from build123d import *

# Parameters (mm, degrees)
SKETCH2_R           = 50
SKETCH2_R_2         = 30
BOSS_EXTRUDE1_DEPTH = 25
SKETCH3_W           = 66
SKETCH3_H           = 13
CUT_EXTRUDE1_DEPTH  = 25


with BuildPart() as part:
    # Sketch2 → Boss-Extrude1 (new body)
    with BuildSketch(Plane(origin=(0, 0, 0), x_dir=(1, 0, 0), z_dir=(0, 1, 0))):
        with Locations(Location((0, 0, 0), (0, 0, 270))):
            Circle(SKETCH2_R)
        with Locations(Location((0, 0, 0), (0, 0, 270))):
            Circle(SKETCH2_R_2, mode=Mode.SUBTRACT)
    extrude(amount=BOSS_EXTRUDE1_DEPTH)

    # Sketch3 → Cut-Extrude1 (cut)
    with BuildSketch(Plane(origin=(0, 25, 0), x_dir=(1, 0, 0), z_dir=(0, 1, 0))):
        with Locations((0, 1.5)):
            Rectangle(SKETCH3_W, SKETCH3_H)
    extrude(amount=-CUT_EXTRUDE1_DEPTH, mode=Mode.SUBTRACT)


solid = part.part
Could you check a few things on this model? Use its own coordinates, in mm. A direction names the side the tool comes from. Give positions to 0.01 mm unless a question says otherwise; leave off trailing zeros. Order: outer loops, then holes, each group sorted by start corner. A loop starts at its lowest first (then second) coordinate and runs counter-clockwise, first axis right, second up.
1. Suppose I cut it at D-D (x = 40). List the corners of the cut face in (y, z) for me, plus the area to 3 significant figures.
2. Suppose I cut it at B-B (z = 0). List the corners of the cut face in (x, y) for me, plus the area to 3 significant figures.
3. Will these pins go through, and if not, where does the flat tip stop? P1, Ø1.7, axis at x = -32, y = 15, coming from the -Z side; P2, Ø2, axis at x = 30, y = 15.5, coming from the +Z side; P3, Ø12, axis at x = -8, y = 15.5, coming from the +Z side; P4, Ø10, axis at x = 26.5, z = -7.5, coming from the +Y side.
4. Suppose I cut it at A-A (x = 0). List the corners of the cut face in (y, z) for me, plus the area to 3 significant figures.
5. For faces 1 (the flat face through (-22, 0, 22)), 2 (the flat face through (-33, 13, -1)), which set-ups out of +Z, -Z, +X, -X, +Y, -Y let a thin tool reach every point of the face, with its end or its side?
6. Suppose I cut it at C-C (y = 21). List the corners of the cut face in (x, z) for me.
7. I need wall thicknesses on L1, parallel to X at y = 18.75, z = 18; L2, parallel to X at y = 21, z = -25.5; L3, parallel to Z at x = 19, y = 19. Which ranges of each line are inside material? Lowest first, please.
8. We'd pull the mould along Z, two halves only. Please class faces 3 (the cylindrical face through (15.02, 12.32, 47.69)), 4 (the flat face through (31, 13, 5)), 5 (the flat face through (-22, 25, 22)): pulls with the +Z half, pulls with the -Z half, needs draft (parallel to the pull), parting line crosses it, or undercut.
Solved:
1. outline: (0, -30) - (25, -30) - (25, 30) - (0, 30) - close
1. area: 1,500 mm2
2. outline: (-50, 0) - (-33, 0) - (-33, 25) - (-50, 25) - close; (33, 0) - (50, 0) - (50, 25) - (33, 25) - close
2. area: 850 mm2
3. P1: stops at z = -39.11
3. P2: stops at z = 40.73
3. P3: stops at z = 49.96
3. P4: stops at y = 25
4. outline: (0, -50) - (25, -50) - (25, -30) - (0, -30) - close; (0, 30) - (25, 30) - (25, 50) - (0, 50) - close
4. area: 1,000 mm2
5. face 1: +Z, -Z, +X, -X, -Y
5. face 2: +Y, -Y
6. outline: circle Ø100 at (0, 0); hole (-33, -8) - (-28.91, -8) arc R30 ccw to (28.91, -8) - (33, -8) - (33, 5) - (29.58, 5) arc R30 ccw to (-29.58, 5) - (-33, 5) - close
7. L1: x = -46.65 to -24, 24 to 46.65
7. L2: x = -43.01 to -15.8, 15.8 to 43.01
7. L3: z = -46.25 to -23.22, 23.22 to 46.25
8. face 3: parting line crosses it
8. face 4: undercut
8. face 5: needs draft
